Autodesk Inventor part; units mm, degrees
ref_plane "YZ Plane" through (0, 0, 0) normal (1, 0, 0) x (0, 1, 0)
ref_plane "XZ Plane" through (0, 0, 0) normal (0, 1, 0) x (-1, 0, 0)
ref_plane "XY Plane" through (0, 0, 0) normal (0, 0, 1) x (1, 0, 0)
sketch "スケッチ1" plane through (0, 0, 0) normal (0, 0, 1) x (1, 0, 0)
  circle A0 centre (0, 0) radius 4
  circle A1 centre (0, 0) radius 8
  circle A2 centre (0, 0) radius 6 construction
  circle A3 centre (0, 6) radius 1.1
  circle A4 centre (-4.2426, 4.2426) radius 1.1
  circle A5 centre (-6, 0) radius 1.1
  circle A6 centre (-4.2426, -4.2426) radius 1.1
  circle A7 centre (0, -6) radius 1.1
  circle A8 centre (4.2426, -4.2426) radius 1.1
  circle A9 centre (6, 0) radius 1.1
  circle A10 centre (4.2426, 4.2426) radius 1.1
  dimension "d2" = 12
  dimension "d0" = 8
  dimension "d1" = 16
  dimension "d3" = 2.2
  dimension "d6" = 360
extrude "押し出し1" add sketch "スケッチ1" along normal blind 3
sketch "スケッチ2" plane through (0, 0, 0) normal (0, 0, -1) x (-1, 0, 0)
  circle A0 centre (-12.8215, -6.6226) radius 1.3
  circle A1 centre (-12.8215, -6.6226) radius 3
  circle A2 centre (0, 0) radius 8
  line L0 (-15.0365, -4.5993) -> (-5.9067, 5.3955)
  line L1 (-12.4536, -9.5999) -> (0.9812, -7.9396)
  circle A3 centre (-4.758, 14.0841) radius 3
  circle A4 centre (-12.8215, -6.6226) radius 1.3 construction
  dimension "d10" = 2.6
  dimension "d11" = 6
extrude "押し出し2" add sketch "スケッチ2" against normal blind 3 contours A1 | A1 L0 A2 L1
sketch "スケッチ3" plane through (0, 0, 3) normal (0, 0, 1) x (1, 0, 0)
  circle A0 centre (0, -6) radius 1.1
  circle A1 centre (0, -6) radius 2
  circle A2 centre (0, 0) radius 4
  circle A3 centre (4.2426, -4.2426) radius 2
  circle A4 centre (6, 0) radius 2
  circle A5 centre (4.2426, 4.2426) radius 2
  circle A6 centre (0, 6) radius 2
  circle A7 centre (-4.2426, 4.2426) radius 2
  circle A8 centre (-6, 0) radius 2
  circle A9 centre (-4.2426, -4.2426) radius 2
  point P0 (0, -4)
  point P1 (-2.8284, -2.8284)
  point P2 (-4, 0)
  point P3 (-2.8284, 2.8284)
  point P4 (0, 4)
  point P5 (2.8284, 2.8284)
  point P6 (4, 0)
  point P7 (2.8284, -2.8284)
  dimension "d15" = 4
  dimension "d18" = 360
extrude "押し出し3" cut sketch "スケッチ3" against normal blind 1.5 contours A0 | A1 | A9 | A8 | A7 | A6 | A5 | A4 | A3 | A2
properties part number "namida" material "アルミニウム 2014-T4"
Geometry: final body of the model. Coordinates: model frame, mm. A direction names the side the tool comes from. Round coordinates to 2 decimals unless told otherwise and drop trailing zeros. Order: outer loops, then holes, each group sorted by start corner. A loop starts at its lowest first (then second) coordinate and runs counter-clockwise, first axis right, second up. Notation, with made-up numbers: (31, -12) -> (51, -12) arc R11 ccw to (51, 7) -> close; hole circle Ø5 at (67.25, 63.5). An arc over 180 degrees is marked (long way). Write each question's results on one line, items separated by ' | '.
Q1. Section query B-B (z = 1). Count the separate pieces of the cut face and the enclosed holes in it, and give its area (3 significant figures).
Response values:
separate pieces: 1 | enclosed holes: 10 | area: 197 mm²
Q2. Pin query (flat end, axial travel): pin 1 Ø3.5 at (x, y) = (0, 6) entering from +Z; pin 2 Ø1.3 at (x, y) = (4.24, -4.24) entering from +Z. Return the tip coordinate at first contact, or that it passes through.
Response values:
pin 1: z = 1.5 | pin 2: through
Q3. Section query C-C (x = 1.75). Output: boundary loops of the cut face in (y, z).
Response values:
outline: (-8.28, 0) -> (-3.6, 0) -> (-3.6, 3) -> (-5.03, 3) -> (-5.03, 1.5) -> (-6.97, 1.5) -> (-6.97, 3) -> (-8.28, 3) -> close; (3.6, 0) -> (7.81, 0) -> (7.81, 3) -> (6.97, 3) -> (6.97, 1.5) -> (5.03, 1.5) -> (5.03, 3) -> (3.6, 3) -> close
Q4. Section query A-A (x = -6). Output: boundary loops of the cut face in (y, z).
Response values:
outline: (-5.29, 0) -> (-1.1, 0) -> (-1.1, 1.5) -> (-2, 1.5) -> (-2, 3) -> (-3.29, 3) -> (-3.29, 1.5) -> (-5.2, 1.5) -> (-5.2, 3) -> (-5.29, 3) -> close; (1.1, 0) -> (5.29, 0) -> (5.29, 3) -> (5.2, 3) -> (5.2, 1.5) -> (3.29, 1.5) -> (3.29, 3) -> (2, 3) -> (2, 1.5) -> (1.1, 1.5) -> close
Q5. Pull-direction query (X, two-part tool) for faces 3 (the face through (5.83, -8.78, 1.48)), 4 (the face through (-3, 3, 1.5)), 5 (the face through (-4, 2, 3)); classes: released by +X, released by -X, zero draft, split by the parting line, or undercut.
Response values:
face 3: released by -X | face 4: undercut | face 5: zero draft
Q6. Ray query, line 1 along Y through (x, z) = (-0.5, 1.3); line 2 along Z through (x, y) = (1.25, -5.75); line 3 along X through (y, z) = (-3.5, 1.15). Return the intervals inside material, ascending.
Response values:
line 1: -8 to -6.98, -5.02 to -3.97, 3.97 to 5.02, 6.98 to 7.98 | line 2: 0 to 1.5 | line 3: -7.19 to -5.05, -3.43 to -1.94, 1.94 to 3.43, 5.05 to 14.03
Q7. Section query D-D (x = 10). Output: boundary loops of the cut face in (y, z).
Response values:
outline: (-9.3, 0) -> (0.91, 0) -> (0.91, 3) -> (-9.3, 3) -> close
Q8. Access query for faces 1 (the face through (0.59, 5.07, 0.74)), 2 (the face through (1, -7, 1.5)). Directions: +Z, -Z, +X, -X, +Y, -Y. A direction counts if a zero-diameter tool reaches every point of the face in a straight line with its end or side. Return the directions, or none.
Response values:
face 1: +Z, -Z | face 2: +Z
